The figure shows three views and two pictorial views of one solid part (mm, origin at its lowest corner). Answer the questions. A direction names the side the tool comes from. Coordinates: 2 decimals unless noted, no trailing zeros. Loops run counter-clockwise (first coordinate to the right, second up) from the corner with the lowest first, then second, coordinate; pieces in that order, holes last. Notation, with made-up numbers: M -14,74.5 L 39,74.5 A26 ccw 39,108.5 Z; hole C 67,-29.75 d5. An arc over 180 degrees is marked long. Return JSON: item names as keys, results as strings. Group by question number.
1. The mould has two halves that part along Z. Classify the marked faces 4, 5 and 6: pulls with the +Z half, pulls with the -Z half, needs draft (parallel to the pull), parting line crosses it, or undercut.
2. Section C-C (x = 66.25) is taken. Write down the section's boundary in (y, z).
3. Section B-B (y = 3.25) is taken. Write down the section's boundary in (x, z).
4. Section D-D (y = 9.25) is taken. Write down the section's boundary in (x, z).
5. Straight lines are drawn through the part: L1, parallel to Z at x = 8.75, y = 4.7; L2, parallel to X at y = 3.8, z = 15; L3, parallel to X at y = 3.5, z = 15. For each, find the intervals that lie inside material, in ascending order. Write a range as from..to.
6. Given P1, Ø5, axis at y = 7.5, z = 8, coming from the -X side; P2, Ø4, axis at x = 29, z = 15, coming from the -Y side; P3, Ø5, axis at x = 65, z = 9.5, coming from the +Y side, each flat-ended and moving along its own axis, determine where each tip first touches the part or whether it passes through.
7. Which of the six approach directions +Z, -Z, +X, -X, +Y, -Y give full straight-line access (tool end or side, diameter ignored) to the marked faces 1, 2 and 3?
8. Section A-A (z = 15) is taken. Write down the section's boundary in (x, y), then the cut area to 3 significant figures.
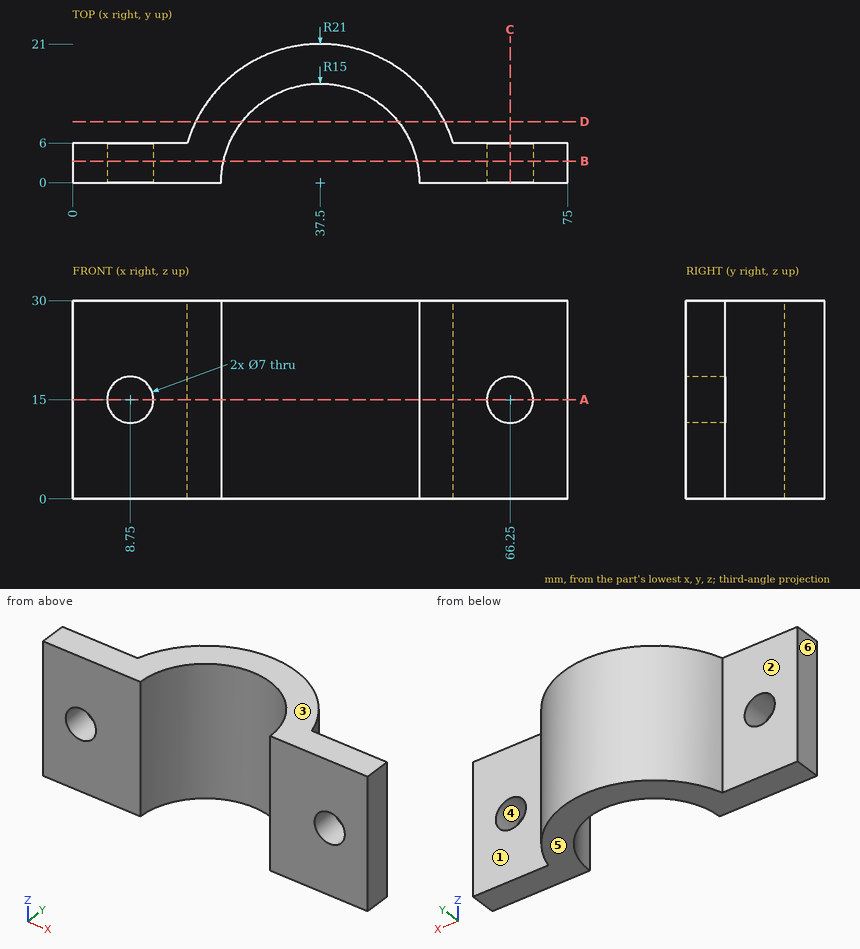
Worked out:
{
 "1": {"face 4": "undercut", "face 5": "pulls with the -Z half", "face 6": "needs draft"},
 "2": {"outline": "M 0,0 L 6,0 L 6,11.5 L 0,11.5 Z; M 0,18.5 L 6,18.5 L 6,30 L 0,30 Z"},
 "3": {"outline": "M 0,0 L 22.86,0 L 22.86,30 L 0,30 Z; M 52.14,0 L 75,0 L 75,30 L 52.14,30 Z; hole C 8.75,15 d7; hole C 66.25,15 d7"},
 "4": {"outline": "M 18.65,0 L 25.69,0 L 25.69,30 L 18.65,30 Z; M 49.31,0 L 56.35,0 L 56.35,30 L 49.31,30 Z"},
 "5": {"L1": "0..11.5, 18.5..30", "L2": "0..5.25, 12.25..22.99, 52.01..62.75, 69.75..75", "L3": "0..5.25, 12.25..22.91, 52.09..62.75, 69.75..75"},
 "6": {"P1": "x = 0", "P2": "y = 10.71", "P3": "y = 6"},
 "7": {"face 1": "+Z, -Z, +X, +Y", "face 2": "+Z, -Z, -X, +Y", "face 3": "+Z, +X, -X, +Y, -Y"},
 "8": {"outline": "M 0,0 L 5.25,0 L 5.25,6 L 0,6 Z; M 12.25,0 L 22.5,0 A15 cw 52.5,0 L 62.75,0 L 62.75,6 L 57.62,6 A21 ccw 17.38,6 L 12.25,6 Z; M 69.75,0 L 75,0 L 75,6 L 69.75,6 Z", "area": "457 mm^2"}
}
